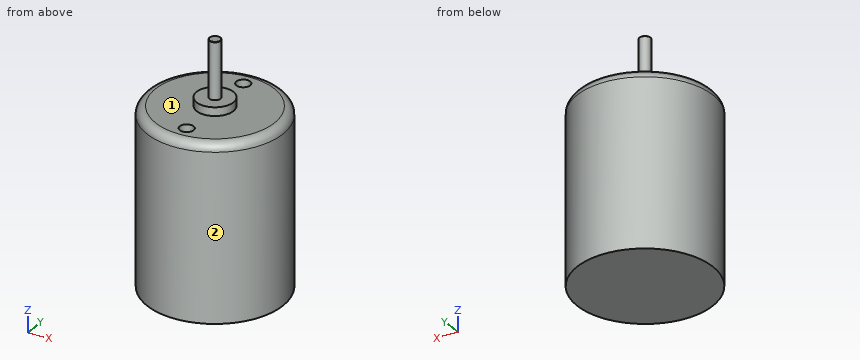
Autodesk Inventor part; units mm, degrees
ref_plane "YZ Plane" through (0, 0, 0) normal (1, 0, 0) x (0, 1, 0)
ref_plane "XZ Plane" through (0, 0, 0) normal (0, 1, 0) x (-1, 0, 0)
ref_plane "XY Plane" through (0, 0, 0) normal (0, 0, 1) x (1, 0, 0)
sketch "スケッチ1" plane through (0, 0, 0) normal (0, 0, 1) x (1, 0, 0)
  circle A0 centre (0, 0) radius 12
  dimension "d0" = 24
extrude "押し出し1" add sketch "スケッチ1" along normal blind 31
sketch "スケッチ2" plane through (0, 0, 31) normal (0, 0, 1) x (1, 0, 0)
  circle A0 centre (0, 0) radius 9.8 construction
  line L0 (0, -16.8) -> (0, 16.8) construction
  circle A1 centre (0, 8.3) radius 1.5
  circle A2 centre (0, -8.3) radius 1.5
  circle A3 centre (0, 0) radius 3.25
  dimension "d3" = 19.6
  dimension "d4" = 3
  dimension "d5" = 3
  dimension "d6" = 6.5
extrude "押し出し2" add sketch "スケッチ2" along normal blind 1.5 contours A3
hole "穴1" at (0, 8.3, 31) at (0, -8.3, 31) direction (0, 0, -1) diameter 2.459 depth 8.8 tip angle 118
fillet "フィレット1" radius 1.5 1 edges at (-12, 0, 31)
sketch "スケッチ3" plane through (0, 0, 32.5) normal (0, 0, 1) x (1, 0, 0)
  circle A0 centre (0, 0) radius 3.25
  circle A1 centre (0, 0) radius 1
  dimension "d17" = 2
extrude "押し出し3" add sketch "スケッチ3" along normal blind 10 contours A1
fillet "フィレット2" radius 0.1 1 edges at (-1, 0, 42.5)
properties part number "tamiya_sporttuned"
The listing builds one solid part. Answer for the finished solid, in the listing's coordinates (mm). Face numbers are marked on the shaded views. A direction names the side the tool comes from. Give positions to 0.01 mm unless a question says otherwise; leave off trailing zeros. Order: outer loops, then holes, each group sorted by start corner. A loop starts at its lowest first (then second) coordinate and runs counter-clockwise, first axis right, second up. Notation, with made-up numbers: (49, 74.25) -> (65, 74.25) arc R28 ccw to (65, 94.25) -> close; hole circle Ø9 at (32, 65.5). An arc over 180 degrees is marked (long way). Answer as a JSON object with one key per item and string values. Group by question number.
Item 1: The part is cut by section D-D on z = 16. Write down the section's boundary in (x, y), and give its area (3 significant figures).
Item 2: Flat-ended cylindrical pins translate along their axes: pin 1 (4 mm diameter, centred on y = -2, z = 36, fed in from -X); pin 2 (4 mm diameter, centred on y = -3.5, z = 13, fed in from -X); pin 3 (6 mm diameter, centred on y = -8.5, z = 19, fed in from +X). Find the tip coordinate at first contact, or state that the pin passes through.
Item 3: The part is cut by section A-A on y = 0. Write down the section's boundary in (x, z).
Item 4: The part is cut by section B-B on z = 32. Write down the section's boundary in (x, y), and give its area (3 significant figures).
Item 5: The part is cut by section C-C on z = 25. Write down the section's boundary in (x, y), and give its area (3 significant figures).
Item 6: Consider L1, parallel to Y at x = 0, z = 29; L2, parallel to X at y = -8.3, z = 26; L3, parallel to Z at x = 6, y = -1.25. Determine where each line is inside the solid, lowest interval first. Write a range as from..to.
Item 7: A tool of negligible diameter and unlimited length cuts with its end or side. For the marked faces 1 and 2, from which of +Z, -Z, +X, -X, +Y, -Y can it reach the whole face along a straight path? Write none if from no direction.
Result set:
{
 "1": {"outline": "circle Ø24 at (0, 0)", "area": "452 mm²"},
 "2": {"pin 1": "x = -1", "pin 2": "x = -11.91", "pin 3": "x = 10.67"},
 "3": {"outline": "(-12, 0) -> (12, 0) -> (12, 29.5) arc R1.5 ccw to (10.5, 31) -> (3.25, 31) -> (3.25, 32.5) -> (1, 32.5) -> (1, 42.4) arc R0.1 ccw to (0.9, 42.5) -> (-0.9, 42.5) arc R0.1 ccw to (-1, 42.4) -> (-1, 32.5) -> (-3.25, 32.5) -> (-3.25, 31) -> (-10.5, 31) arc R1.5 ccw to (-12, 29.5) -> close"},
 "4": {"outline": "circle Ø6.5 at (0, 0)", "area": "33.2 mm²"},
 "5": {"outline": "circle Ø24 at (0, 0); hole circle Ø2.46 at (0, -8.3); hole circle Ø2.46 at (0, 8.3)", "area": "443 mm²"},
 "6": {"L1": "-12..-9.53, -7.07..7.07, 9.53..12", "L2": "-8.67..-1.23, 1.23..8.67", "L3": "0..31"},
 "7": {"face 1": "+Z", "face 2": "+Z, -Z"}
}
